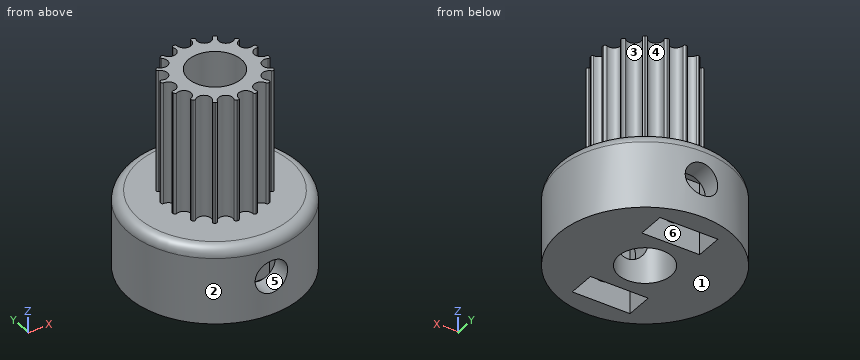
```python
from build123d import *

# Parameters (mm, degrees)
SKETCH_1_R          = 8.5
SKETCH_1_R_2        = 2.6
EXTRUDE_1_DEPTH     = 7.5
FILLET_1_R          = 1
SKETCH_6_R          = 2.6
EXTRUDE_2_DEPTH     = 12
SKETCH_4_R          = 1.6
CUT_EXTRUDE_1_DEPTH = 23.907422415
SKETCH_5_W          = 5.7
SKETCH_5_H          = 2.7
CUT_EXTRUDE_2_DEPTH = 7.05


with BuildPart() as part:
    # 草图1 → 凸台-拉伸1 (new body)
    with BuildSketch(Plane.XY):
        Circle(SKETCH_1_R)
        Circle(SKETCH_1_R_2, mode=Mode.SUBTRACT)
    extrude(amount=EXTRUDE_1_DEPTH)

    # 圆角1
    fillet_1_edges = [part.edges().sort_by_distance(p)[0] for p in [
        (-8.5, 0, 7.5),
    ]]
    fillet(fillet_1_edges, radius=FILLET_1_R)

    # 草图6 → 凸台-拉伸2 (add)
    with BuildSketch(Plane.XY.offset(7.5)):
        with BuildLine():
            ThreePointArc((-0.888859814, 4.755603807), (-0.943838819, 4.744998169), (-0.998691399, 4.733756947))
            ThreePointArc((-0.998691399, 4.733756947), (-1.108499785, 4.649297568), (-1.111229207, 4.510791906))
            ThreePointArc((-1.111229207, 4.510791906), (-1.480203512, 3.573527394), (-2.403853838, 3.975369253))
            ThreePointArc((-2.403853838, 3.975369253), (-2.503722124, 4.071377553), (-2.641090177, 4.053453098))
            ThreePointArc((-2.641090177, 4.053453098), (-2.687825553, 4.022615211), (-2.734200899, 3.991238503))
            ThreePointArc((-2.734200899, 3.991238503), (-2.803329414, 3.871186362), (-2.752847249, 3.742179311))
            ThreePointArc((-2.752847249, 3.742179311), (-2.735059458, 2.735059458), (-3.742179311, 2.752847249))
            ThreePointArc((-3.742179311, 2.752847249), (-3.871186362, 2.803329414), (-3.991238503, 2.734200899))
            ThreePointArc((-3.991238503, 2.734200899), (-4.022615211, 2.687825553), (-4.053453098, 2.641090177))
            ThreePointArc((-4.053453098, 2.641090177), (-4.071377553, 2.503722124), (-3.975369253, 2.403853838))
            ThreePointArc((-3.975369253, 2.403853838), (-3.573527394, 1.480203512), (-4.510791906, 1.111229207))
            ThreePointArc((-4.510791906, 1.111229207), (-4.649297568, 1.108499785), (-4.733756947, 0.998691399))
            ThreePointArc((-4.733756947, 0.998691399), (-4.744998169, 0.943838819), (-4.755603807, 0.888859814))
            ThreePointArc((-4.755603807, 0.888859814), (-4.719595366, 0.755088889), (-4.592677324, 0.699563409))
            ThreePointArc((-4.592677324, 0.699563409), (-3.867958179, 0), (-4.592677324, -0.699563409))
            ThreePointArc((-4.592677324, -0.699563409), (-4.719595366, -0.755088889), (-4.755603807, -0.888859814))
            ThreePointArc((-4.755603807, -0.888859814), (-4.744998169, -0.943838819), (-4.733756947, -0.998691399))
            ThreePointArc((-4.733756947, -0.998691399), (-4.649297568, -1.108499785), (-4.510791906, -1.111229207))
            ThreePointArc((-4.510791906, -1.111229207), (-3.573527394, -1.480203512), (-3.975369253, -2.403853838))
            ThreePointArc((-3.975369253, -2.403853838), (-4.071377553, -2.503722124), (-4.053453098, -2.641090177))
            ThreePointArc((-4.053453098, -2.641090177), (-4.022615211, -2.687825553), (-3.991238503, -2.734200899))
            ThreePointArc((-3.991238503, -2.734200899), (-3.871186362, -2.803329414), (-3.742179311, -2.752847249))
            ThreePointArc((-3.742179311, -2.752847249), (-2.735059458, -2.735059458), (-2.752847249, -3.742179311))
            ThreePointArc((-2.752847249, -3.742179311), (-2.803329414, -3.871186362), (-2.734200899, -3.991238503))
            ThreePointArc((-2.734200899, -3.991238503), (-2.687825553, -4.022615211), (-2.641090177, -4.053453098))
            ThreePointArc((-2.641090177, -4.053453098), (-2.503722124, -4.071377553), (-2.403853838, -3.975369253))
            ThreePointArc((-2.403853838, -3.975369253), (-1.480203512, -3.573527394), (-1.111229207, -4.510791906))
            ThreePointArc((-1.111229207, -4.510791906), (-1.108499785, -4.649297568), (-0.998691399, -4.733756947))
            ThreePointArc((-0.998691399, -4.733756947), (-0.943838819, -4.744998169), (-0.888859814, -4.755603807))
            ThreePointArc((-0.888859814, -4.755603807), (-0.755088889, -4.719595366), (-0.699563409, -4.592677324))
            ThreePointArc((-0.699563409, -4.592677324), (0, -3.867958179), (0.699563409, -4.592677324))
            ThreePointArc((0.699563409, -4.592677324), (0.755088889, -4.719595366), (0.888859814, -4.755603807))
            ThreePointArc((0.888859814, -4.755603807), (0.943838819, -4.744998169), (0.998691399, -4.733756947))
            ThreePointArc((0.998691399, -4.733756947), (1.108499785, -4.649297568), (1.111229207, -4.510791906))
            ThreePointArc((1.111229207, -4.510791906), (1.480203512, -3.573527394), (2.403853838, -3.975369253))
            ThreePointArc((2.403853838, -3.975369253), (2.503722124, -4.071377553), (2.641090177, -4.053453098))
            ThreePointArc((2.641090177, -4.053453098), (2.687825553, -4.022615211), (2.734200899, -3.991238503))
            ThreePointArc((2.734200899, -3.991238503), (2.803329414, -3.871186362), (2.752847249, -3.742179311))
            ThreePointArc((2.752847249, -3.742179311), (2.735059458, -2.735059458), (3.742179311, -2.752847249))
            ThreePointArc((3.742179311, -2.752847249), (3.871186362, -2.803329414), (3.991238503, -2.734200899))
            ThreePointArc((3.991238503, -2.734200899), (4.022615211, -2.687825553), (4.053453098, -2.641090177))
            ThreePointArc((4.053453098, -2.641090177), (4.071377553, -2.503722124), (3.975369253, -2.403853838))
            ThreePointArc((3.975369253, -2.403853838), (3.573527394, -1.480203512), (4.510791906, -1.111229207))
            ThreePointArc((4.510791906, -1.111229207), (4.649297568, -1.108499785), (4.733756947, -0.998691399))
            ThreePointArc((4.733756947, -0.998691399), (4.744998169, -0.943838819), (4.755603807, -0.888859814))
            ThreePointArc((4.755603807, -0.888859814), (4.719595366, -0.755088889), (4.592677324, -0.699563409))
            ThreePointArc((4.592677324, -0.699563409), (3.867958179, 0), (4.592677324, 0.699563409))
            ThreePointArc((4.592677324, 0.699563409), (4.719595366, 0.755088889), (4.755603807, 0.888859814))
            ThreePointArc((4.755603807, 0.888859814), (4.744998169, 0.943838819), (4.733756947, 0.998691399))
            ThreePointArc((4.733756947, 0.998691399), (4.649297568, 1.108499785), (4.510791906, 1.111229207))
            ThreePointArc((4.510791906, 1.111229207), (3.573527394, 1.480203512), (3.975369253, 2.403853838))
            ThreePointArc((3.975369253, 2.403853838), (4.071377553, 2.503722124), (4.053453098, 2.641090177))
            ThreePointArc((4.053453098, 2.641090177), (4.022615211, 2.687825553), (3.991238503, 2.734200899))
            ThreePointArc((3.991238503, 2.734200899), (3.871186362, 2.803329414), (3.742179311, 2.752847249))
            ThreePointArc((3.742179311, 2.752847249), (2.735059458, 2.735059458), (2.752847249, 3.742179311))
            ThreePointArc((2.752847249, 3.742179311), (2.803329414, 3.871186362), (2.734200899, 3.991238503))
            ThreePointArc((2.734200899, 3.991238503), (2.687825553, 4.022615211), (2.641090177, 4.053453098))
            ThreePointArc((2.641090177, 4.053453098), (2.503722124, 4.071377553), (2.403853838, 3.975369253))
            ThreePointArc((2.403853838, 3.975369253), (1.480203512, 3.573527394), (1.111229207, 4.510791906))
            ThreePointArc((1.111229207, 4.510791906), (1.108499785, 4.649297568), (0.998691399, 4.733756947))
            ThreePointArc((0.998691399, 4.733756947), (0.943838819, 4.744998169), (0.888859814, 4.755603807))
            ThreePointArc((0.888859814, 4.755603807), (0.755088889, 4.719595366), (0.699563409, 4.592677324))
            ThreePointArc((0.699563409, 4.592677324), (0, 3.867958179), (-0.699563409, 4.592677324))
            ThreePointArc((-0.699563409, 4.592677324), (-0.755088889, 4.719595366), (-0.888859814, 4.755603807))
        make_face()
        Circle(SKETCH_6_R, mode=Mode.SUBTRACT)
    extrude(amount=EXTRUDE_2_DEPTH)

    # 草图4 → 切除-拉伸1 (cut, symmetric)
    with BuildSketch(Plane(origin=(0, 0, 0), x_dir=(1, 0, 0), z_dir=(0, 1, 0))):
        with Locations(Location((0, -3.75, 0), (0, 0, 270))):
            Circle(SKETCH_4_R)
    cut_extrude_1 = extrude(amount=CUT_EXTRUDE_1_DEPTH, both=True, mode=Mode.SUBTRACT)

    # 草图5 → 切除-拉伸2 (cut)
    with BuildSketch(Plane(origin=(0, 0, 0), x_dir=(-1, 0, 0), z_dir=(0, 0, -1))):
        with Locations((0, 5.15)):
            Rectangle(SKETCH_5_W, SKETCH_5_H)
    cut_extrude_2 = extrude(amount=-CUT_EXTRUDE_2_DEPTH, mode=Mode.SUBTRACT)

    # 镜向1: 切除-拉伸1, 切除-拉伸2 across plane
    add(cut_extrude_1.mirror(Plane.ZX), mode=Mode.SUBTRACT)
    add(cut_extrude_2.mirror(Plane.ZX), mode=Mode.SUBTRACT)


solid = part.part
```
Work out the finished part from the listing and answer in its coordinate system (mm). Face numbers are marked on the shaded views. A direction names the side the tool comes from. Coordinates: 2 decimals unless noted, no trailing zeros. Write each loop counter-clockwise with the first axis right and the second up, starting at its lowest first coordinate (ties: lowest second). Pieces come first, ordered by that corner, then holes.
Q1. A cutting plane is placed at C-C, the plane z = 3.75. Give the vertices of the cut face in (x, y), then the cut area to 3 significant figures.
Q2. A cutting plane is placed at B-B, the plane z = 1.75. Give the vertices of the cut face in (x, y), then the cut area to 3 significant figures.
Q3. A cutting plane is placed at A-A, the plane y = 0. Give the vertices of the cut face in (x, z), then the cut area to 3 significant figures.
Q4. Each of these flat-tipped pins is pushed along its axis until it touches: pin 1 Ø2 at (x, z) = (-4.5, 3.5) entering from -Y; pin 2 Ø1 at (x, z) = (-5, 5.5) entering from -Y; pin 3 Ø3 at (x, z) = (-1, 4) entering from -Y; pin 4 Ø3 at (x, z) = (0, 3.75) entering from -Y. Where does it stop, or does it pass through?
Q5. Which of the six approach directions +Z, -Z, +X, -X, +Y, -Y give full straight-line access (tool end or side, diameter ignored) to the marked faces 4, 5 and 6?
Q6. Determine the mould class of the marked faces 1, 2 and 3 for opening direction X: released by +X, released by -X, zero draft, split by the parting line, or undercut.
Q7. Find the intervals of material crossed by line 1 (X direction, y = 3.75, z = 15.75); line 2 (Z direction, x = 0, y = 3.4); line 3 (Z direction, x = 0, y = -7.2), in increasing order.
Findings below:
1. outline: (-2.85, -6.5) - (-2.85, -3.8) - (-1.6, -3.8) - (-1.6, -2.05) arc R2.6 cw to (-1.6, 2.05) - (-1.6, 3.8) - (-2.85, 3.8) - (-2.85, 6.5) - (-1.6, 6.5) - (-1.6, 8.35) arc R8.5 ccw to (-1.6, -8.35) - (-1.6, -6.5) - close; (1.6, -8.35) arc R8.5 ccw to (1.6, 8.35) - (1.6, 6.5) - (2.85, 6.5) - (2.85, 3.8) - (1.6, 3.8) - (1.6, 2.05) arc R2.6 cw to (1.6, -2.05) - (1.6, -3.8) - (2.85, -3.8) - (2.85, -6.5) - (1.6, -6.5) - close
1. area: 154 mm2
2. outline: circle Ø17 at (0, 0); hole (-2.85, -6.5) - (2.85, -6.5) - (2.85, -3.8) - (-2.85, -3.8) - close; hole (-2.85, 3.8) - (2.85, 3.8) - (2.85, 6.5) - (-2.85, 6.5) - close; hole circle Ø5.2 at (0, 0)
2. area: 175 mm2
3. outline: (-8.5, 0) - (-2.6, 0) - (-2.6, 19.5) - (-3.87, 19.5) - (-3.87, 7.5) - (-7.5, 7.5) arc R1 ccw to (-8.5, 6.5) - close; (2.6, 0) - (8.5, 0) - (8.5, 6.5) arc R1 ccw to (7.5, 7.5) - (3.87, 7.5) - (3.87, 19.5) - (2.6, 19.5) - close
3. area: 119 mm2
4. pin 1: stops at y = -7.75
4. pin 2: stops at y = -7.21
4. pin 3: stops at y = -8.49
4. pin 4: passes through
5. face 4: +Z
5. face 5: +Y, -Y
5. face 6: -Z
6. face 1: zero draft
6. face 2: split by the parting line
6. face 3: undercut
7. line 1: x = -2.76 to -2.27, -1.23 to 1.23, 2.27 to 2.76
7. line 2: z = 0 to 2.15, 5.35 to 19.5
7. line 3: z = 0 to 2.15, 5.35 to 7.5
